Can you work these out from the drawing? Everything is in mm from the part's minimum corner. Round coordinates to 2 decimals unless told otherwise and drop trailing zeros. Loops run counter-clockwise (first coordinate to the right, second up) from the corner with the lowest first, then second, coordinate; pieces in that order, holes last. Notation, with made-up numbers: (-11, -0.5) -> (24, -0.5) arc R28 cw to (24, 23.5) -> close; hole circle Ø6 at (17, 29.25). An arc over 180 degrees is marked (long way). One line per item, written item: value.
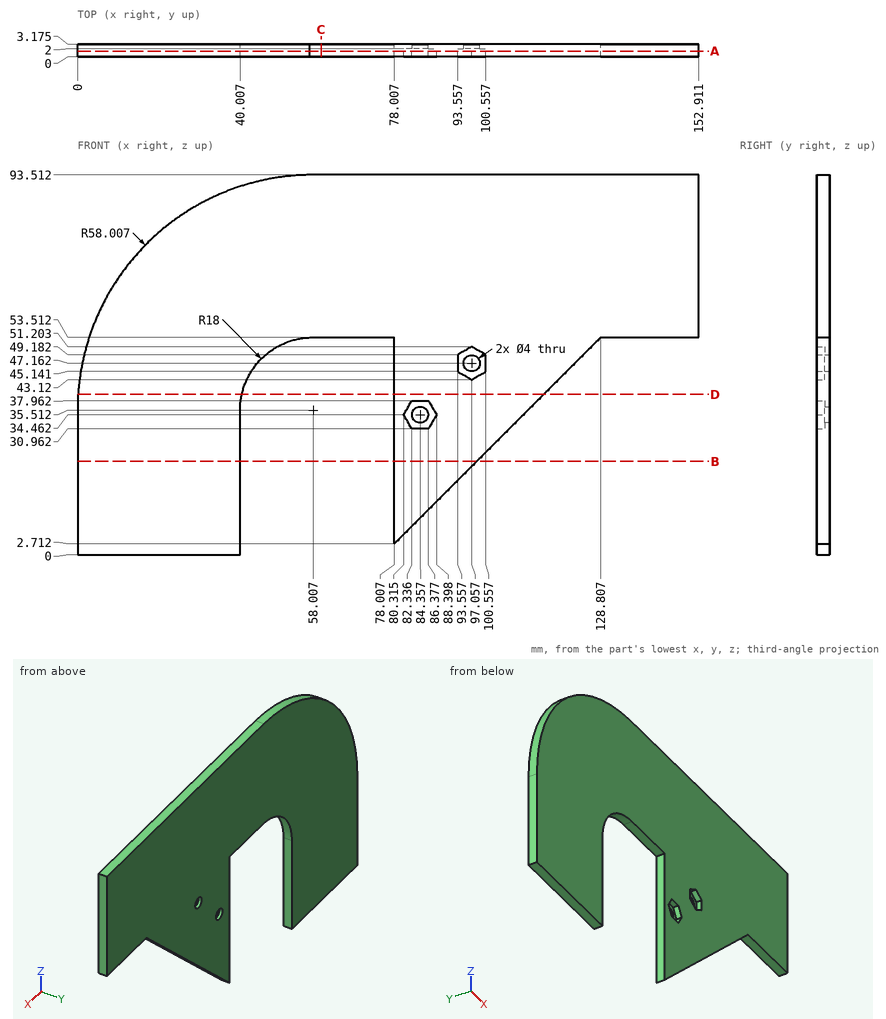
Item 1: If we section it at C-C on x = 60: List the corners of the cut face in (y, z) for me (1 decimal).
Output:
outline: (0, 53.5) -> (3.2, 53.5) -> (3.2, 93.5) -> (0, 93.5) -> close
Item 2: If we section it at A-A on y = 1.45: List the corners of the cut face in (x, z) for me (1 decimal), plus the area to 3 significant figures.
Output:
outline: (0, 0) -> (40, 0) -> (40, 35.5) arc R18 cw to (58, 53.5) -> (78, 53.5) -> (78, 2.7) -> (128.8, 53.5) -> (152.9, 53.5) -> (152.9, 93.5) -> (57.1, 93.5) arc R58 ccw to (0, 35.5) -> close; hole (80.3, 34.5) -> (82.3, 31) -> (86.4, 31) -> (88.4, 34.5) -> (86.4, 38) -> (82.3, 38) -> close; hole (93.6, 45.1) -> (97.1, 43.1) -> (100.6, 45.1) -> (100.6, 49.2) -> (97.1, 51.2) -> (93.6, 49.2) -> close
area: 8,810 mm²
Item 3: I need wall thicknesses on line 1 (X direction, y = 0.6, z = 45) (1 decimal); line 2 (Z direction, x = 69, y = 2.75); line 3 (X direction, y = 1, z = 25.5) (1 decimal). Which ranges of each line are inside material? Lowest first, please. Write a range as from..to.
Output:
line 1: x = 0.8..42.7, 78..93.8, 100.3..120.3
line 2: z = 53.51..93.51
line 3: x = 0..40, 78..100.8
Item 4: Will these pins go through, and if not, where does the flat tip stop? pin 1 Ø1.6 at (x, y) = (137.5, 2) entering from -Z; pin 2 Ø1 at (y, z) = (2, 19.5) entering from +X (1 decimal); pin 3 Ø1.6 at (x, y) = (84, 1) entering from -Z (1 decimal); pin 4 Ø2 at (x, z) = (96.5, 47.5) entering from -Y.
Output:
pin 1: stops at z = 53.51
pin 2: stops at x = 95.3
pin 3: stops at z = 7.9
pin 4: passes through
Item 5: If we section it at B-B on z = 23: List the corners of the cut face in (x, y) for me (1 decimal).
Output:
outline: (0, 0) -> (40, 0) -> (40, 3.2) -> (0, 3.2) -> close; (78, 0) -> (98.3, 0) -> (98.3, 3.2) -> (78, 3.2) -> close
Item 6: If we section it at D-D on z = 39.5: List the corners of the cut face in (x, y) for me (1 decimal).
Output:
outline: (0.1, 0) -> (40.5, 0) -> (40.5, 3.2) -> (0.1, 3.2) -> close; (78, 0) -> (114.8, 0) -> (114.8, 3.2) -> (78, 3.2) -> close
